```python
from build123d import *

# Parameters (mm, degrees)
F0_R     = 20
F1_DEPTH = 20
F2_W     = 3.1
F2_H     = 7.1
F2_W_2   = 7.1
F2_H_2   = 3.1
F3_DEPTH = 15
F4_W     = 50
F4_H     = 50
F5_DEPTH = 5


with BuildPart() as f1:
    # F0 (on Top) → F1 (new body)
    with BuildSketch(Plane.XY):
        Circle(F0_R)
    extrude(amount=F1_DEPTH)

    # F2 (on face) → F3 (cut)
    with BuildSketch(Plane(origin=(0, 0, 0), x_dir=(1, 0, 0), z_dir=(0, 0, -1))):
        with Locations((0, -10.55)):
            Rectangle(F2_W, F2_H)
        with Locations((8.55, 6.55)):
            Rectangle(F2_W_2, F2_H_2)
        with Locations((-8.55, 6.55)):
            Rectangle(F2_W_2, F2_H_2)
    extrude(amount=-F3_DEPTH, mode=Mode.SUBTRACT)

    # F4 (on face) → F5 (join)
    with BuildSketch(Plane.XY.offset(20)):
        Rectangle(F4_W, F4_H)
    extrude(amount=F5_DEPTH)


solid = f1.part
```
CAD build for the part. Positions are in the model's coordinates, mm. A direction names the side the tool comes from. Round coordinates to 2 decimals unless told otherwise and drop trailing zeros. Loops run counter-clockwise (first coordinate to the right, second up) from the corner with the lowest first, then second, coordinate; pieces in that order, holes last. Notation, with made-up numbers: M 22.25,-30.5 L 75.25,-30.5 A33 cw 75.25,3.5 Z; hole C -14,-6 d10. An arc over 180 degrees is marked long. Use a Markdown table: item, result. Add a question column.
(1) Cut at C-C (y = 0). Give the cut face in (x, z), and give its area (3 significant figures).
(2) Drill centre lines: line 1 (Z direction, x = -19.5, y = -16); line 2 (Y direction, x = -11, z = 1.75); line 3 (Y direction, x = -10.5, z = 4.75). Where is each one in solid material? Low to high.
(3) Cut at D-D (x = 0). Give the cut face in (y, z).
(4) Flat gauge pins, fed straight in: pin 1 (3.5 mm diameter, centred on x = 0, z = 9, fed in from -Y); pin 2 (8 mm diameter, centred on y = 1.5, z = 13, fed in from +X); pin 3 (1 mm diameter, centred on y = -7, z = 4.5, fed in from +X). Where does each tip first touch, or does it go through?
(5) Which spindle directions (+Z, -Z, +X, -X, +Y, -Y) get a long thin tool onto all of the face, cutting with end or side? Do faces 1 (the face through (0, 25, 22)), 2 (the face through (-5, -7, 7)). Say none if no direction does.
(6) Pull direction X, two halves, no side cores. Call faces 3 (the face through (0, 14.1, 7)), 4 (the face through (9, -7, 15)), 5 (the face through (-17, 11, 20)), 6 (the face through (-4.336, -19.524, 9.86)): +X half, -X half, draft (parallel to the pull), parting line (faces both ways), or undercut.
(7) Cut at A-A (x = 16). Give the cut face in (y, z).
(8) Cut at B-B (z = 1.5). Give the cut face in (x, y).
Geometry says:
| question | item | result |
|---|---|---|
| 1 | outline | M -25,20 L -20,20 L -20,0 L 20,0 L 20,20 L 25,20 L 25,25 L -25,25 Z |
| 1 | area | 1,050 mm² |
| 2 | line 1 | z = 20 to 25 |
| 2 | line 2 | y = -16.7 to -8.1, -5 to 16.7 |
| 2 | line 3 | y = -17.02 to -8.1, -5 to 17.02 |
| 3 | outline | M -25,20 L -20,20 L -20,0 L 7,0 L 7,15 L 14.1,15 L 14.1,0 L 20,0 L 20,20 L 25,20 L 25,25 L -25,25 Z |
| 4 | pin 1 | stops at y = -20 |
| 4 | pin 2 | stops at x = 20 |
| 4 | pin 3 | stops at x = 18.91 |
| 5 | face 1 | +Z, -Z, +X, -X, +Y |
| 5 | face 2 | -Z |
| 6 | face 3 | undercut |
| 6 | face 4 | undercut |
| 6 | face 5 | draft |
| 6 | face 6 | parting line |
| 7 | outline | M -25,20 L -12,20 L -12,0 L 12,0 L 12,20 L 25,20 L 25,25 L -25,25 Z |
| 8 | outline | C 0,0 d40; hole M -12.1,-8.1 L -5,-8.1 L -5,-5 L -12.1,-5 Z; hole M -1.55,7 L 1.55,7 L 1.55,14.1 L -1.55,14.1 Z; hole M 5,-8.1 L 12.1,-8.1 L 12.1,-5 L 5,-5 Z |
